Input: part model. Units: mm. Frame: model coordinates. Coordinates: 2 decimals unless noted, no trailing zeros. Write each loop counter-clockwise with the first axis right and the second up, starting at its lowest first coordinate (ties: lowest second). Pieces come first, ordered by that corner, then holes. Notation, with made-up numbers: M 39.25,20 L 50.25,20 A21 ccw 50.25,56 Z; hole C -18.5,74 d2. An arc over 180 degrees is marked long. Write each question's results on one line, items separated by ' | '. Start each with the question number.
1. Ray query, probe 1 along Y at (x, z) = (-11.6, -97); probe 2 along Y at (x, z) = (-10.5, -118.5). Return the intervals inside material, ascending.
2. First-contact query: pin 1 (1.6 mm diameter, centred on y = 14, z = -119, fed in from +X); pin 2 (3.5 mm diameter, centred on x = 3, z = -50.5, fed in from -Y); pin 3 (0.6 mm diameter, centred on y = 13.5, z = -84.5, fed in from -X); pin 4 (0.6 mm diameter, centred on y = -14.5, z = -100, fed in from +X). Flat tips, straight axial feed; report the tip coordinate or a pass-through.
3. Section query A-A, the plane x = 11.6. Output: boundary loops of the cut face in (y, z), and give its area (3 significant figures).
4. Section query C-C, the plane z = -68. Count the separate pieces of the cut face and the enclosed holes in it, and give its area (3 significant figures).
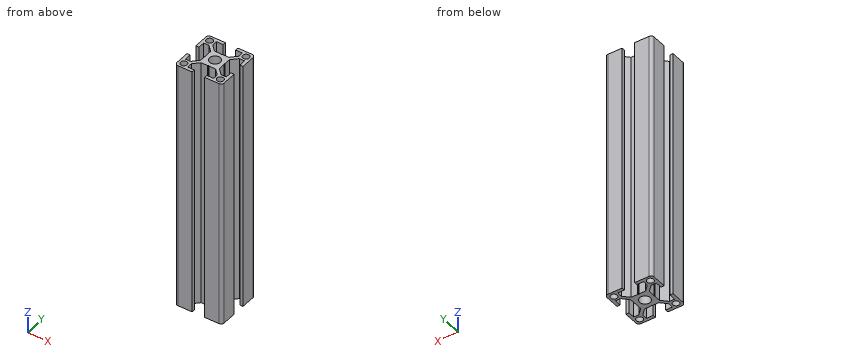
Autodesk Inventor part; units mm, degrees
ref_plane "C1_XY" through (0, 0, 0) normal (0, 0, 1) x (1, 0, 0)
ref_plane "C1_YZ" through (0, 0, 0) normal (1, 0, 0) x (0, 1, 0)
ref_plane "C1_ZX" through (0, 0, 0) normal (0, 1, 0) x (0, 0, 1)
sketch "Sketch_1" plane through (0, 0, 0) normal (0, 0, 1) x (1, 0, 0)
  line L0 (-15, 4) -> (-13, 4)
  line L1 (-13, 4) -> (-13, 8.25)
  line L2 (-13, 8.25) -> (-9.6642, 8.25)
  line L3 (-9.6642, 8.25) -> (-6, 4.5858)
  line L4 (-6, 4.5858) -> (-6, 0.5196)
  line L5 (-6, 0.5196) -> (-5.7, 0)
  line L6 (-5.7, 0) -> (-6, -0.5196)
  line L7 (-6, -0.5196) -> (-6, -4.5858)
  line L8 (-6, -4.5858) -> (-9.6642, -8.25)
  line L9 (-9.6642, -8.25) -> (-13, -8.25)
  line L10 (-13, -8.25) -> (-13, -4)
  line L11 (-13, -4) -> (-15, -4)
  line L12 (-15, -4) -> (-15, -13)
  arc A0 (-15, -13) -> (-13, -15) centre (-13, -13) ccw
  line L13 (-13, -15) -> (-4, -15)
  line L14 (-4, -15) -> (-4, -13)
  line L15 (-4, -13) -> (-8.25, -13)
  line L16 (-8.25, -13) -> (-8.25, -9.6642)
  line L17 (-8.25, -9.6642) -> (-4.5858, -6)
  line L18 (-4.5858, -6) -> (-0.5196, -6)
  line L19 (-0.5196, -6) -> (0, -5.7)
  line L20 (0, -5.7) -> (0.5196, -6)
  line L21 (0.5196, -6) -> (4.5858, -6)
  line L22 (4.5858, -6) -> (8.25, -9.6642)
  line L23 (8.25, -9.6642) -> (8.25, -13)
  line L24 (8.25, -13) -> (4, -13)
  line L25 (4, -13) -> (4, -15)
  line L26 (4, -15) -> (13, -15)
  arc A1 (13, -15) -> (15, -13) centre (13, -13) ccw
  line L27 (15, -13) -> (15, -4)
  line L28 (15, -4) -> (13, -4)
  line L29 (13, -4) -> (13, -8.25)
  line L30 (13, -8.25) -> (9.6642, -8.25)
  line L31 (9.6642, -8.25) -> (6, -4.5858)
  line L32 (6, -4.5858) -> (6, -0.5196)
  line L33 (6, -0.5196) -> (5.7, 0)
  line L34 (5.7, 0) -> (6, 0.5196)
  line L35 (6, 0.5196) -> (6, 4.5858)
  line L36 (6, 4.5858) -> (9.6642, 8.25)
  line L37 (9.6642, 8.25) -> (13, 8.25)
  line L38 (13, 8.25) -> (13, 4)
  line L39 (13, 4) -> (15, 4)
  line L40 (15, 4) -> (15, 13)
  arc A2 (15, 13) -> (13, 15) centre (13, 13) ccw
  line L41 (13, 15) -> (4, 15)
  line L42 (4, 15) -> (4, 13)
  line L43 (4, 13) -> (8.25, 13)
  line L44 (8.25, 13) -> (8.25, 9.6642)
  line L45 (8.25, 9.6642) -> (4.5858, 6)
  line L46 (4.5858, 6) -> (0.5196, 6)
  line L47 (0.5196, 6) -> (0, 5.7)
  line L48 (0, 5.7) -> (-0.5196, 6)
  line L49 (-0.5196, 6) -> (-4.5858, 6)
  line L50 (-4.5858, 6) -> (-8.25, 9.6642)
  line L51 (-8.25, 9.6642) -> (-8.25, 13)
  line L52 (-8.25, 13) -> (-4, 13)
  line L53 (-4, 13) -> (-4, 15)
  line L54 (-4, 15) -> (-13, 15)
  arc A3 (-13, 15) -> (-15, 13) centre (-13, 13) ccw
  line L55 (-15, 13) -> (-15, 4)
extrude "Extrusion1" add sketch "Sketch_1" against normal blind 159
sketch "Sketch2" plane through (0, 0, -159) normal (0, 0, -1) x (-1, 0, 0)
  point P0 (0, 0)
hole "Hole1" at (0, 0, -159) direction (0, 0, 1) diameter 6.8 depth 159
sketch "Sketch3" plane through (0, 0, -159) normal (0, 0, -1) x (-1, 0, 0)
  point P0 (-11.6, 11.6)
hole "Hole2" at (11.6, 11.6, -159) direction (0, 0, 1) diameter 4.2 depth 159
pattern_linear "Rectangular Pattern1" count 2 spacing 23.2 along (-1, 0, 0) count 2 spacing 23.2 along (0, -1, 0) of "Hole2"
ref_plane "C1_XY" through (0, 0, 0) normal (0, 0, 1) x (1, 0, 0)
ref_plane "C1_YZ" through (0, 0, 0) normal (1, 0, 0) x (0, 1, 0)
ref_plane "C1_ZX" through (0, 0, 0) normal (0, 1, 0) x (0, 0, 1)
ref_plane "to_frame_cap1_XY" through (0, 0, 0) normal (0, 0, 1) x (1, 0, 0)
ref_plane "to_frame_cap1_YZ" through (0, 0, 0) normal (1, 0, 0) x (0, 1, 0)
ref_plane "to_frame_cap1_ZX" through (0, 0, 0) normal (0, 1, 0) x (0, 0, 1)
ref_plane "to_frame_cap2_XY" through (0, 0, -159) normal (0, 0, -1) x (1, 0, 0)
ref_plane "to_frame_cap2_YZ" through (0, 0, -159) normal (1, 0, 0) x (0, -1, 0)
ref_plane "to_frame_cap2_ZX" through (0, 0, -159) normal (0, -1, 0) x (0, 0, -1)
properties part number "HFS6-3030-159"
Answer:
1) probe 1: -15 to -13.7, -9.5 to -8.25, 8.25 to 9.5, 13.7 to 15 | probe 2: -15 to -13.39, -9.81 to -8.25, 8.25 to 9.81, 13.39 to 15
2) pin 1: x = 14.99 | pin 2: y = -15 | pin 3: x = -14.99 | pin 4: x = 14.6
3) outline: M -15,-159 L -13.7,-159 L -13.7,0 L -15,0 Z; M -9.5,-159 L -8.25,-159 L -8.25,0 L -9.5,0 Z; M 8.25,-159 L 9.5,-159 L 9.5,0 L 8.25,0 Z; M 13.7,-159 L 15,-159 L 15,0 L 13.7,0 Z | area: 811 mm^2
4) separate pieces: 1 | enclosed holes: 5 | area: 332 mm^2
